from build123d import *

# Parameters (mm, degrees)
RESSALTO_EXTRUS_O1_DEPTH = 2
CORTE_EXTRUS_O1_DEPTH    = 3


with BuildPart() as part:
    # Esboço1 → Ressalto-extrusão1 (new body)
    with BuildSketch(Plane(origin=(0, 0, 0), x_dir=(1, 0, 0), z_dir=(0, 1, 0))):
        with BuildLine():
            Line((-69.067178301, 27.690493718), (-21.84180506, 33.612777476))
            ThreePointArc((-21.84180506, 33.612777476), (-21.220866866, 33.671045747), (-20.597504043, 33.690493718))
            Line((-20.597504043, 33.690493718), (0, 33.690493718))
            Line((0, 33.690493718), (0, -23.309506282))
            Line((0, -23.309506282), (-28.608479685, -23.309506282))
            ThreePointArc((-28.608479685, -23.309506282), (-31.695562463, -22.821073972), (-34.481079048, -21.403490265))
            Line((-34.481079048, -21.403490265), (-69.067178301, 3.690493718))
            Line((-69.067178301, 3.690493718), (-69.067178301, 8.690493718))
            Line((-69.067178301, 8.690493718), (-71.567178301, 8.690493718))
            Line((-71.567178301, 8.690493718), (-71.567178301, 22.690493718))
            Line((-71.567178301, 22.690493718), (-69.067178301, 22.690493718))
            Line((-69.067178301, 22.690493718), (-69.067178301, 27.690493718))
        make_face()
    ressalto_extrus_o1 = extrude(amount=RESSALTO_EXTRUS_O1_DEPTH)

    # Espelhar1: Ressalto-extrusão1 across plane
    add(ressalto_extrus_o1.mirror(Plane(origin=(0, 2, 23.309506282), x_dir=(0, 0, 1), z_dir=(-1, 0, 0))))

    # Esboço2 → Corte-extrusão1 (cut, through all)
    with BuildSketch(Plane(origin=(0, 2, 0), x_dir=(1, 0, 0), z_dir=(0, 1, 0))):
        with BuildLine():
            Line((-48.432821699, 18.690493718), (56.567178301, 18.690493718))
            ThreePointArc((56.567178301, 18.690493718), (57.274285082, 18.397600499), (57.567178301, 17.690493718))
            Line((57.567178301, 17.690493718), (57.567178301, 13.190493718))
            ThreePointArc((57.567178301, 13.190493718), (57.274285082, 12.483386937), (56.567178301, 12.190493718))
            Line((56.567178301, 12.190493718), (-2.932821699, 12.190493718))
            Line((-2.932821699, 12.190493718), (-2.932821699, -16.809506282))
            Line((-2.932821699, -16.809506282), (-9.432821699, -16.809506282))
            Line((-9.432821699, -16.809506282), (-9.432821699, 12.190493718))
            Line((-9.432821699, 12.190493718), (-48.432821699, 12.190493718))
            ThreePointArc((-48.432821699, 12.190493718), (-49.13992848, 12.483386937), (-49.432821699, 13.190493718))
            Line((-49.432821699, 13.190493718), (-49.432821699, 17.690493718))
            ThreePointArc((-49.432821699, 17.690493718), (-49.13992848, 18.397600499), (-48.432821699, 18.690493718))
        make_face()
    extrude(amount=-CORTE_EXTRUS_O1_DEPTH, mode=Mode.SUBTRACT)


solid = part.part
Source: CAD feature listing. Evaluate the final solid. Frame: model axes, mm. Round coordinates to 2 decimals unless told otherwise and drop trailing zeros. Order: outer loops, then holes, each group sorted by start corner. A loop starts at its lowest first (then second) coordinate and runs counter-clockwise, first axis right, second up. Notation, with made-up numbers: (-9, 60.25) -> (43, 60.25) arc R12 cw to (43, 74.25) -> close; hole circle Ø9 at (-38, -27). An arc over 180 degrees is marked (long way). Answer as CSV lines item,"result".
Item 1: Line query: L1, parallel to Z at x = 9, y = 0.3; L2, parallel to X at y = 1.8, z = -11.5; L3, parallel to X at y = 0.35, z = -15. Output: solid intervals per line, ascending.
A:
L1,"-33.69 to -18.69, -12.19 to 23.31"
L2,"-71.57 to -9.43, -2.93 to 71.57"
L3,"-71.57 to -49.43, 57.57 to 71.57"
Item 2: Section C-C, the plane z = -10. Return loops of the section in (x, y).
A:
outline,"(-71.57, 0) -> (-9.43, 0) -> (-9.43, 2) -> (-71.57, 2) -> close; (-2.93, 0) -> (71.57, 0) -> (71.57, 2) -> (-2.93, 2) -> close"
Item 3: Section D-D, the plane x = -54. Return loops of the section in (y, z), plus the area to 3 significant figures.
A:
outline,"(0, -29.58) -> (2, -29.58) -> (2, 7.24) -> (0, 7.24) -> close"
area,"73.6 mm²"
Item 4: Section A-A, the plane x = 8.5. Return loops of the section in (y, z).
A:
outline,"(0, -33.69) -> (2, -33.69) -> (2, -18.69) -> (0, -18.69) -> close; (0, -12.19) -> (2, -12.19) -> (2, 23.31) -> (0, 23.31) -> close"
Item 5: Pin query (flat end, axial travel): pin 1 Ø1 at (x, y) = (-70.5, 0.5) entering from +Z; pin 2 Ø0.6 at (x, y) = (70, 1.5) entering from -Z; pin 3 Ø0.6 at (x, y) = (-34, 1) entering from -Z. Return the tip coordinate at first contact, or that it passes through.
A:
pin 1,"z = -8.69"
pin 2,"z = -22.69"
pin 3,"z = -32.13"
